Source: three-view drawing plus pictorial views. Frame: mm from the lowest corner of the part. Round coordinates to 2 decimals unless told otherwise and drop trailing zeros. Order: outer loops, then holes, each group sorted by start corner. A loop starts at its lowest first (then second) coordinate and runs counter-clockwise, first axis right, second up. Notation, with made-up numbers: M 64.5,61 L 97.5,61 A10 ccw 97.5,69 Z; hole C 35,-5 d6. An arc over 180 degrees is marked long. Return JSON: item names as keys, results as strings. Group by question number.
Q1. Cut plane A-A on z = 5. Output: boundary loops of the cut face in (x, y).
Q2. Cut plane C-C on z = 53. Output: boundary loops of the cut face in (x, y), and give its area (3 significant figures).
Q3. Ray query, probe 1 along Z at (x, y) = (41.5, 2.8); probe 2 along X at (y, z) = (1.1, 7); probe 3 along Z at (x, y) = (12.5, 1.9). Return the intervals inside material, ascending.
Q4. Contact query for flat-ended pins moving along their axis: pin 1 (8 mm diameter, centred on x = 57.5, z = 45.5, fed in from -Y); pin 2 (0.5 mm diameter, centred on y = 1, z = 41, fed in from +X); pin 3 (0.5 mm diameter, centred on x = 42.5, y = 1, fed in from -Z). Output: stop coordinate, or through.
Q5. Cut plane B-B on x = 56. Output: boundary loops of the cut face in (y, z).
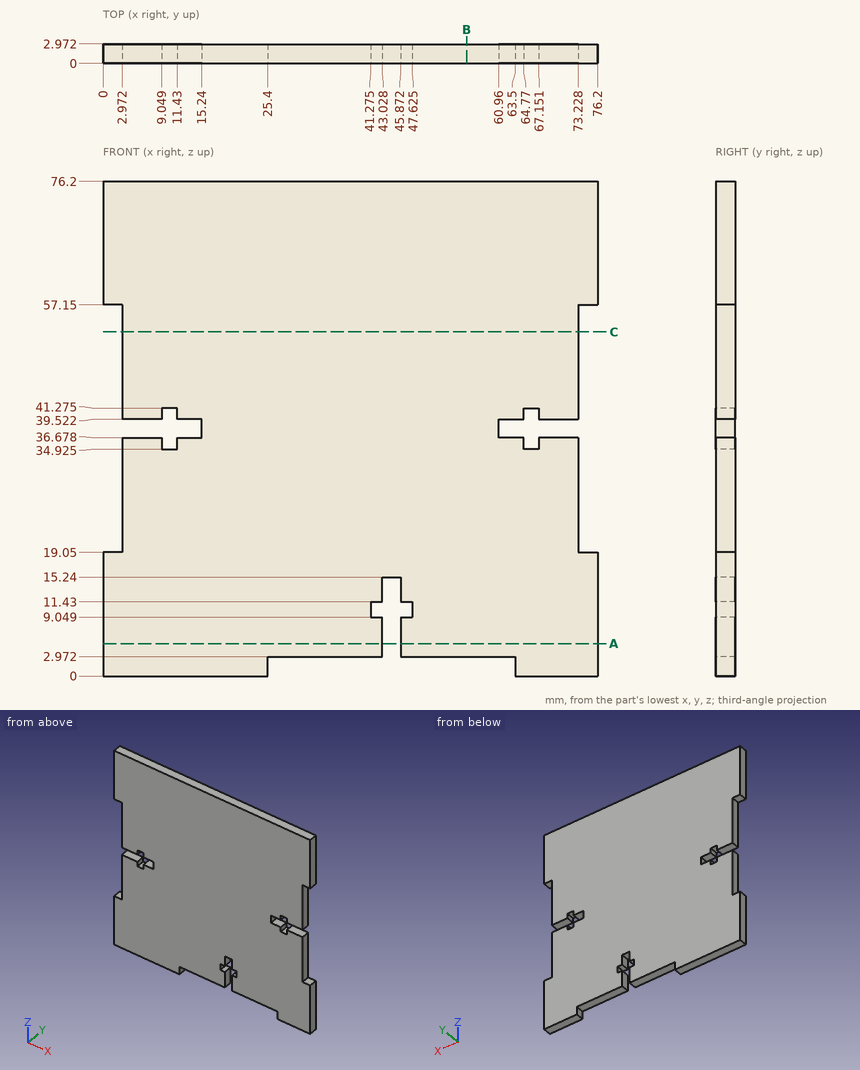
Result sheet:
{
 "1": {"outline": "M 0,0 L 43.03,0 L 43.03,2.97 L 0,2.97 Z; M 45.87,0 L 76.2,0 L 76.2,2.97 L 45.87,2.97 Z"},
 "2": {"outline": "M 2.97,0 L 73.23,0 L 73.23,2.97 L 2.97,2.97 Z", "area": "209 mm²"},
 "3": {"probe 1": "z = 2.97 to 9.05, 11.43 to 76.2", "probe 2": "x = 0 to 43.03, 45.87 to 76.2", "probe 3": "z = 0 to 36.68, 39.52 to 76.2"},
 "4": {"pin 1": "stops at y = 0", "pin 2": "stops at x = 73.23", "pin 3": "stops at z = 2.97"},
 "5": {"outline": "M 0,2.97 L 2.97,2.97 L 2.97,76.2 L 0,76.2 Z"}
}
